Verification items for the finished model (mm, model axes). Round coordinates to 2 decimals unless told otherwise and drop trailing zeros. Write each loop counter-clockwise with the first axis right and the second up, starting at its lowest first coordinate (ties: lowest second). Pieces come first, ordered by that corner, then holes. Notation, with made-up numbers: M -27.75,52 L -20.75,52 A33 cw -20.75,90 Z; hole C -23,12.25 d5. An arc over 180 degrees is marked long. One line per item, written item: value. Start each with the question number.
Item 1: Section check A-A, the plane x = 2.4. Record the cut outline in (y, z), then the cut area to 3 significant figures.
Item 2: Thickness scan on probe 1 along Z at (x, y) = (0.65, 147.5); probe 2 along Z at (x, y) = (0.4, 45.5). Record the ranges inside material, lowest first. Write a range as from..to.
Item 3: Gauge pin test, flat end, axial feed: pin 1 (1.5 mm diameter, centred on x = 2.5, y = 178.5, fed in from +Z). Record the tip position at first contact, or that the pin passes through.
Item 4: Section check B-B, the plane z = 47. Record the cut outline in (x, y) (3 decimals), then the cut area to 3 significant figures.
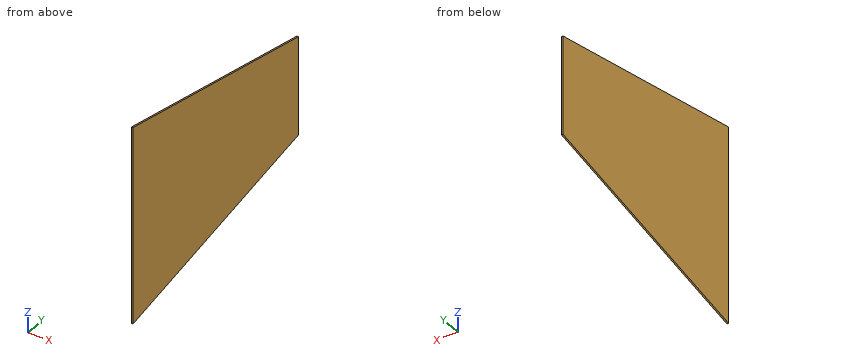
Autodesk Inventor part; units mm, degrees
ref_plane "YZ Plane" through (0, 0, 0) normal (1, 0, 0) x (0, 1, 0)
ref_plane "XZ Plane" through (0, 0, 0) normal (0, 1, 0) x (-1, 0, 0)
ref_plane "XY Plane" through (0, 0, 0) normal (0, 0, 1) x (1, 0, 0)
sketch "Sketch1" plane through (0, 0, 0) normal (1, 0, 0) x (0, 1, 0)
  line L0 (0, 0) -> (0, 406.4)
  line L1 (0, 0) -> (0, 203.2)
  line L2 (0, 203.2) -> (457.2, 203.2) construction
  line L3 (497.7363, 304.8) -> (497.7363, 101.6)
  line L4 (497.7363, 304.8) -> (0, 406.4)
  line L5 (497.7363, 101.6) -> (0, 0)
  dimension "d0" = 406.4
  dimension "d4" = 203.2
  dimension "d5" = 203.2
  dimension "d11" = 101.6
  dimension "d12" = 101.6
  dimension "d14" = 508
  dimension "d15" = 497.7363
extrude "Extrusion1" add sketch "Sketch1" along normal blind 3.175
properties part number "Polycarb Front Pannel" material "Polycarbonate, Clear"
Response values:
1. outline: M 0,0 L 497.74,101.6 L 497.74,304.8 L 0,406.4 Z
1. area: 152,000 mm2
2. probe 1: z = 30.11..376.29
2. probe 2: z = 9.29..397.11
3. pin 1: stops at z = 370.12
4. outline: M 0,0 L 3.175,0 L 3.175,230.252 L 0,230.252 Z
4. area: 731 mm2
